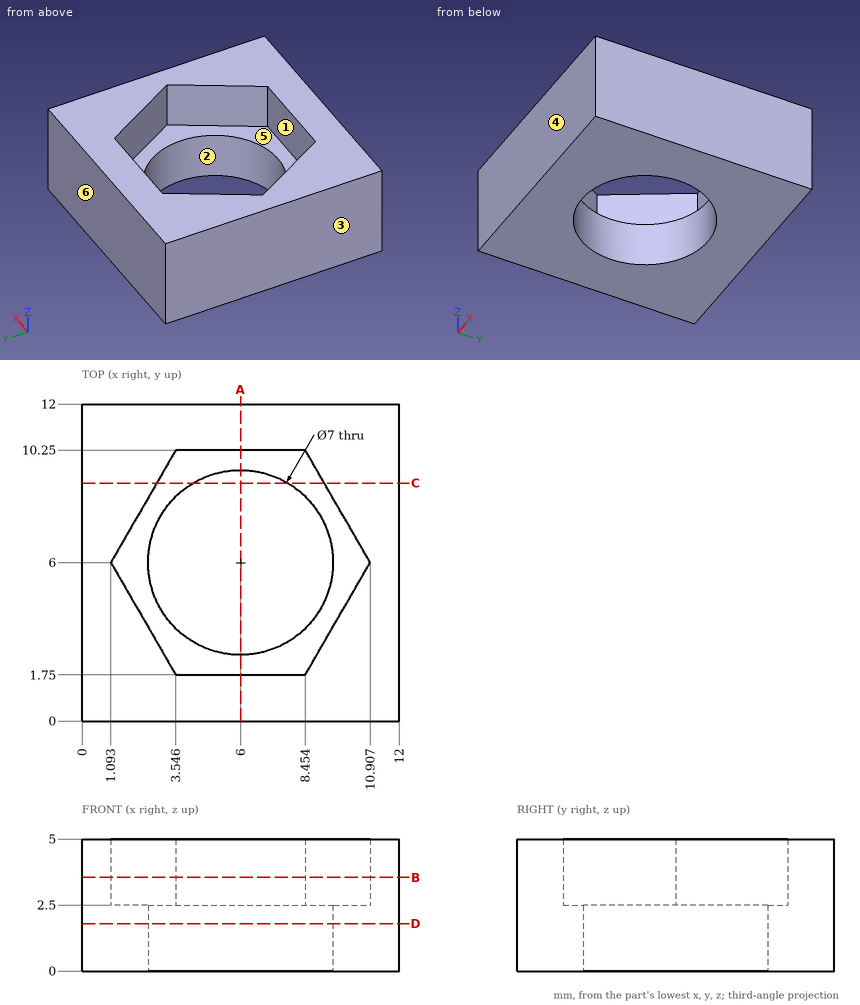
The figure shows three views and two pictorial views of one solid part (mm, origin at its lowest corner). Answer the questions. A direction names the side the tool comes from. Round coordinates to 2 decimals unless told otherwise and drop trailing zeros. Loops run counter-clockwise (first coordinate to the right, second up) from the corner with the lowest first, then second, coordinate; pieces in that order, holes last. Notation, with made-up numbers: M 14,30.25 L 39,30.25 A16 cw 39,61.25 Z; hole C 33.5,80.5 d6. An arc over 180 degrees is marked long. Write each question's results on one line, items separated by ' | '. Start each with the question number.
1) Find section C-C on y = 9. Write down the section's boundary in (x, z) (1 decimal), plus the area to 3 significant figures.
2) Determine the mould class of the marked faces 3, 4, 5 and 6 for opening direction Y: pulls with the +Y half, pulls with the -Y half, needs draft (parallel to the pull), parting line crosses it, or undercut.
3) Which of the six approach directions +Z, -Z, +X, -X, +Y, -Y give full straight-line access (tool end or side, diameter ignored) to the marked faces 1 and 2?
4) Find section B-B on z = 3.55. Write down the section's boundary in (x, y).
5) This flat-tipped pin is pushed along its axis until it touches: pin 1 (1.2 mm diameter, centred on x = 5.5, z = 4, fed in from -Y). Where does it stop, or does it pass through?
6) Find section D-D on z = 1.8. Write down the section's boundary in (x, y).
7) Straight lines are drawn through the part: probe 1 along Y at (x, z) = (6, 1.3); probe 2 along Y at (x, z) = (5.25, 3.7); probe 3 along Z at (x, y) = (4.5, 10). For each, find the intervals that lie inside material, in ascending order.
8) Find section A-A on x = 6. Write down the section's boundary in (y, z).
Final values:
1) outline: M 0,0 L 4.2,0 L 4.2,2.5 L 2.8,2.5 L 2.8,5 L 0,5 Z; M 7.8,0 L 12,0 L 12,5 L 9.2,5 L 9.2,2.5 L 7.8,2.5 Z | area: 35.1 mm²
2) face 3: needs draft | face 4: pulls with the -Y half | face 5: undercut | face 6: pulls with the +Y half
3) face 1: +Z | face 2: +Z, -Z
4) outline: M 0,0 L 12,0 L 12,12 L 0,12 Z; hole M 1.09,6 L 3.55,1.75 L 8.45,1.75 L 10.91,6 L 8.45,10.25 L 3.55,10.25 Z
5) pin 1: y = 0
6) outline: M 0,0 L 12,0 L 12,12 L 0,12 Z; hole C 6,6 d7
7) probe 1: 0 to 2.5, 9.5 to 12 | probe 2: 0 to 1.75, 10.25 to 12 | probe 3: 0 to 2.5
8) outline: M 0,0 L 2.5,0 L 2.5,2.5 L 1.75,2.5 L 1.75,5 L 0,5 Z; M 9.5,0 L 12,0 L 12,5 L 10.25,5 L 10.25,2.5 L 9.5,2.5 Z
